```python
from build123d import *

# Parameters (mm, degrees)
SKETCH1_R           = 1
BOSS_EXTRUDE1_DEPTH = 5
SKETCH2_R           = 5.5
CUT_EXTRUDE1_DEPTH  = 3
SKETCH3_R           = 1.5
CUT_EXTRUDE2_DEPTH  = 82.737384348
SKETCH4_W           = 32
SKETCH4_H           = 20
SKETCH4_R           = 1
SKETCH4_W_2         = 22
SKETCH4_H_2         = 8
BOSS_EXTRUDE2_DEPTH = 5
CUT_EXTRUDE3_DEPTH  = 1.5


with BuildPart() as part:
    # Sketch1 → Boss-Extrude1 (new body)
    with BuildSketch(Plane.XY):
        with BuildLine():
            Line((-16, 0), (-16, 80))
            Line((-16, 80), (16, 80))
            Line((16, 80), (16, 0))
            ThreePointArc((16, 0), (0, -16), (-16, 0))
        make_face()
        Circle(SKETCH1_R, mode=Mode.SUBTRACT)
    extrude(amount=BOSS_EXTRUDE1_DEPTH)

    # Sketch2 → Cut-Extrude1 (cut)
    with BuildSketch(Plane(origin=(0, 0, 0), x_dir=(-1, 0, 0), z_dir=(0, 0, -1))):
        Circle(SKETCH2_R)
    extrude(amount=-CUT_EXTRUDE1_DEPTH, mode=Mode.SUBTRACT)

    # Sketch3 → Cut-Extrude2 (cut, through all)
    with BuildSketch(Plane.XY.offset(5)):
        with Locations((-11, 75)):
            Circle(SKETCH3_R)
        with Locations((11, 75)):
            Circle(SKETCH3_R)
        with Locations((-11, 30)):
            Circle(SKETCH3_R)
        with Locations((11, 30)):
            Circle(SKETCH3_R)
    extrude(amount=-CUT_EXTRUDE2_DEPTH, mode=Mode.SUBTRACT)

    # Sketch4 → Boss-Extrude2 (add)
    with BuildSketch(Plane.XY.offset(5)):
        with Locations((0, 90)):
            Rectangle(SKETCH4_W, SKETCH4_H)
        with Locations((-13.5, 95.8)):
            Circle(SKETCH4_R, mode=Mode.SUBTRACT)
        with Locations((13.5, 95.8)):
            Circle(SKETCH4_R, mode=Mode.SUBTRACT)
        with Locations((-13.5, 87.8)):
            Circle(SKETCH4_R, mode=Mode.SUBTRACT)
        with Locations((13.5, 87.8)):
            Circle(SKETCH4_R, mode=Mode.SUBTRACT)
        with Locations((0, 89.5)):
            Rectangle(SKETCH4_W_2, SKETCH4_H_2, mode=Mode.SUBTRACT)
    extrude(amount=-BOSS_EXTRUDE2_DEPTH)

    # Sketch5 → Cut-Extrude3 (cut)
    with BuildSketch(Plane.XY):
        Polygon((-8.113248654, 75), (-9.556624327, 77.5), (-12.443375673, 77.5), (-13.886751346, 75), (-12.443375673, 72.5), (-9.556624327, 72.5), align=None)
        Polygon((8.113248654, 75), (9.556624327, 72.5), (12.443375673, 72.5), (13.886751346, 75), (12.443375673, 77.5), (9.556624327, 77.5), align=None)
        Polygon((8.113248654, 30), (9.556624327, 27.5), (12.443375673, 27.5), (13.886751346, 30), (12.443375673, 32.5), (9.556624327, 32.5), align=None)
        Polygon((-8.113248654, 30), (-9.556624327, 32.5), (-12.443375673, 32.5), (-13.886751346, 30), (-12.443375673, 27.5), (-9.556624327, 27.5), align=None)
    extrude(amount=CUT_EXTRUDE3_DEPTH, mode=Mode.SUBTRACT)


solid = part.part
```
Could you check a few things on this model? Use its own coordinates, in mm. A direction names the side the tool comes from. Round coordinates to 2 decimals unless told otherwise and drop trailing zeros. Loops run counter-clockwise (first coordinate to the right, second up) from the corner with the lowest first, then second, coordinate; pieces in that order, holes last. Notation, with made-up numbers: M -20.5,-19 L 35.5,-19 A24 cw 35.5,0 Z; hole C -24,13.25 d6. An arc over 180 degrees is marked long. Answer as CSV lines item,"result".
1) Imagine slicing it at B-B on x = 0. List the corners of the cut face in (y, z) for me.
From the geometry:
outline,"M -16,0 L -5.5,0 L -5.5,3 L -1,3 L -1,5 L -16,5 Z; M 1,3 L 5.5,3 L 5.5,0 L 85.5,0 L 85.5,5 L 1,5 Z; M 93.5,0 L 100,0 L 100,5 L 93.5,5 Z"
2) If I drill on probe 1 along X at (y, z) = (95.8, 1.1); probe 2 along X at (y, z) = (75, 2.7); probe 3 along X at (y, z) = (93, 1.5), over which ranges is the centre line in solid material (lowest first)?
From the geometry:
probe 1,"-16 to -14.5, -12.5 to 12.5, 14.5 to 16"
probe 2,"-16 to -12.5, -9.5 to 9.5, 12.5 to 16"
probe 3,"-16 to -11, 11 to 16"
3) Imagine slicing it at C-C on z = 4.1. Count the separate pieces of the cut face and the enclosed holes in it, and give its area (3 significant figures).
From the geometry:
separate pieces,"1"
enclosed holes,"10"
area,"3,380 mm^2"
4) For pin 1 Ø1.5 at (x, y) = (-11.5, 30) entering from -Z; pin 2 Ø2 at (x, z) = (-8, 2) entering from -Y; pin 3 Ø1.6 at (x, z) = (11.5, 0.5) entering from -Y; pin 4 Ø1.5 at (x, z) = (-11, 3) entering from -Y, each with a flat end and sliding along its axis, tell me the tip position at first contact or that it passes through.
From the geometry:
pin 1,"through"
pin 2,"y = -14.39"
pin 3,"y = -11.9"
pin 4,"y = -12.29"
5) Imagine slicing it at A-A on y = 92. List the corners of the cut face in (x, z) for me.
From the geometry:
outline,"M -16,0 L -11,0 L -11,5 L -16,5 Z; M 11,0 L 16,0 L 16,5 L 11,5 Z"
6) Which directions (+Z, -Z, +X, -X, +Y, -Y) give clear straight access to the entire face, cutting with the end or side of a thin tool? Please do faces 5 (the flat face through (-9.76, 31.15, 1.5)), 6 (the flat face through (-11, 89, 3)), 7 (the flat face through (16, 49, 3)).
From the geometry:
face 5,"-Z"
face 6,"+Z, -Z"
face 7,"+Z, -Z, +X, +Y, -Y"
7) We'd pull the mould along X, two halves only. Please class faces 1 (the flat face through (0, 43, 5)), 2 (the cylindrical face through (9.89, 31.01, 3.27)), 3 (the flat face through (-16, 49, 3)), 4 (the cylindrical face through (0, -16, 2)): released by +X, released by -X, zero draft, split by the parting line, or undercut.
From the geometry:
face 1,"zero draft"
face 2,"undercut"
face 3,"released by -X"
face 4,"split by the parting line"
